```python
from build123d import *

# Parameters (mm, degrees)
LOFT2_DEPTH = 35
LOFT2_DRAFT = 15.9453959
SHELL1_T    = -3


# Read off the part's stored shape, not the designer's step: Loft2
with BuildPart() as part:
    # Loft2 outline → Loft2 (with draft: the straight prism first)
    with BuildSketch(Plane.XY.offset(70)):
        Polygon((39.192235936, -105), (42, -93.768943744), (42, 93.532311637), (29.559693491, 135), (-29.559693491, 135), (-42, 93.532311637), (-42, -93.768943744), (-39.192235936, -105), align=None)
    extrude(amount=-LOFT2_DEPTH)
    # Loft2: the draft: its side faces are tilted about the plane it starts from
    loft2_sides = [part.faces().sort_by_distance(p)[0] for p in [
        (40.596117968, -99.384471872, 52.5),
        (42, -0.118316053, 52.5),
        (35.779846746, 114.266155819, 52.5),
        (0, 135, 52.5),
        (-35.779846746, 114.266155818, 52.5),
        (-42, -0.118316053, 52.5),
        (-40.596117968, -99.384471872, 52.5),
        (0, -105, 52.5),
    ]]
    draft(loft2_sides, Plane.XY.offset(70), LOFT2_DRAFT)

    # Shell1
    shell1_openings = [part.faces().sort_by_distance(p)[0] for p in [
        (0, 12.225404098, 35),
    ]]
    offset(amount=SHELL1_T, openings=shell1_openings, kind=Kind.INTERSECTION)


solid = part.part
```
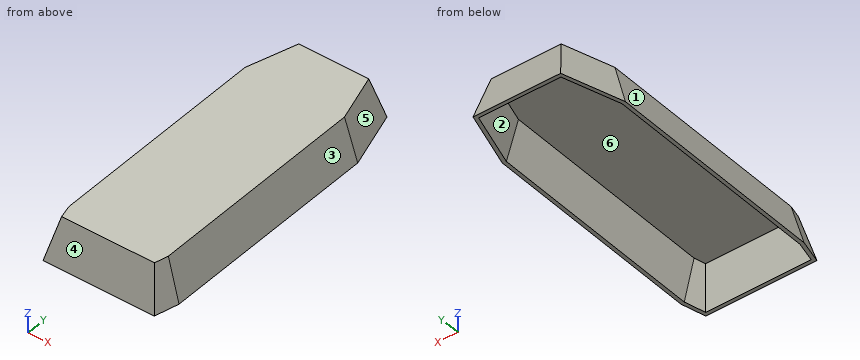
Design review of the part built by this model. Coordinates are the model's own, in mm. Face numbers are marked on the shaded views. A direction names the side the tool comes from. Round coordinates to 2 decimals unless told otherwise and drop trailing zeros. Write each loop counter-clockwise with the first axis right and the second up, starting at its lowest first coordinate (ties: lowest second). Pieces come first, ordered by that corner, then holes.
Item 1: We need section C-C on x = -20. Write out the cut boundary in (y, z), and give its area (3 significant figures).
Item 2: For probe 1 along Z at (x, y) = (-10, -90); probe 2 along X at (y, z) = (122, 56); probe 3 along X at (y, z) = (100.5, 56), list the stretches that pass through material, from the lowest coordinate up.
Item 3: We need section B-B on z = 62. Write out the cut boundary in (x, y), and give its area (3 significant figures).
Item 4: The part is to be moulded in two halves that separate along Y. For the marked faces 3, 4, 5 and 6, say which applies: +Y half, -Y half, draft (parallel to the pull), parting line (faces both ways), or undercut.
Item 5: Clearance check with flat-ended pins moving along their axes: pin 1 Ø8 at (y, z) = (-17.5, 60.5) entering from -X; pin 2 Ø1.5 at (x, y) = (-29, -16) entering from -Z; pin 3 Ø1.5 at (x, z) = (30, 51) entering from +Y. State where each tip first meets the part, or that it passes through.
Item 6: We need section D-D on z = 50.5. Write out the cut boundary in (x, y) (3 decimals), and give its area (3 significant figures).
Item 7: We need section A-A on y = -1.5. Write out the cut boundary in (x, z).
Item 8: For the marked faces 1 and 2, list the 3-axis set-ups (+Z, -Z, +X, -X, +Y, -Y) from which the entire face can be reached by the end or side of a thin tool; tool diameter is ignored.
Returned:
1. outline: (-115, 35) - (-111.88, 35) - (-102.74, 67) - (132.74, 67) - (141.88, 35) - (145, 35) - (135, 70) - (-105, 70) - close
1. area: 922 mm2
2. probe 1: z = 67 to 70
2. probe 2: x = -37.64 to -34.38, 34.38 to 37.64
2. probe 3: x = -44.09 to -40.83, 40.83 to 44.09
3. outline: (-44.29, -94.05) - (-40.98, -107.29) - (40.98, -107.29) - (44.29, -94.05) - (44.29, 93.87) - (31.26, 137.29) - (-31.26, 137.29) - (-44.29, 93.87) - close; hole (-41.17, -93.67) - (-38.54, -104.17) - (38.54, -104.17) - (41.17, -93.67) - (41.17, 93.41) - (28.94, 134.17) - (-28.94, 134.17) - (-41.17, 93.41) - close
3. area: 1,960 mm2
4. face 3: draft
4. face 4: -Y half
4. face 5: +Y half
4. face 6: undercut
5. pin 1: stops at x = -45.86
5. pin 2: stops at z = 67
5. pin 3: stops at y = 140.64
6. outline: (-47.571, -94.455) - (-43.542, -110.571) - (43.542, -110.571) - (47.571, -94.455) - (47.571, 94.35) - (33.705, 140.571) - (-33.705, 140.571) - (-47.571, 94.35) - close; hole (-44.451, -94.071) - (-41.106, -107.451) - (41.106, -107.451) - (44.451, -94.071) - (44.451, 93.892) - (31.384, 137.451) - (-31.384, 137.451) - (-44.451, 93.892) - close
6. area: 2,030 mm2
7. outline: (-52, 35) - (-48.88, 35) - (-39.74, 67) - (39.74, 67) - (48.88, 35) - (52, 35) - (42, 70) - (-42, 70) - close
8. face 1: +Z, -X, +Y, -Y
8. face 2: -Z
